from build123d import *

# Parameters (mm, degrees)
SKETCH_1_R          = 2.1
EXTRUDE_1_DEPTH     = 3
SKETCH_2_R          = 1.6
SKETCH_2_R_2        = 8
CUT_EXTRUDE_1_DEPTH = 3
CUT_EXTRUDE_2_DEPTH = 3
CUT_EXTRUDE_3_DEPTH = 3


with BuildPart() as part:
    # 草图1 → 凸台-拉伸1 (new body)
    with BuildSketch(Plane.XY):
        with BuildLine():
            Line((10, 0), (140, 0))
            ThreePointArc((140, 0), (147.071067812, -2.928932188), (150, -10))
            Line((150, -10), (150, -70))
            ThreePointArc((150, -70), (147.071067812, -77.071067812), (140, -80))
            Line((140, -80), (10, -80))
            ThreePointArc((10, -80), (2.928932188, -77.071067812), (0, -70))
            Line((0, -70), (0, -10))
            ThreePointArc((0, -10), (2.928932188, -2.928932188), (10, 0))
        make_face()
        with Locations((8, -8)):
            Circle(SKETCH_1_R, mode=Mode.SUBTRACT)
        with Locations(Location((8, -72, 0), (0, 0, 180))):
            Circle(SKETCH_1_R, mode=Mode.SUBTRACT)
        with Locations((142, -72)):
            Circle(SKETCH_1_R, mode=Mode.SUBTRACT)
        with Locations(Location((142, -8, 0), (0, 0, 180))):
            Circle(SKETCH_1_R, mode=Mode.SUBTRACT)
    extrude(amount=EXTRUDE_1_DEPTH)

    # 草图2 → 切除-拉伸1 (cut)
    with BuildSketch(Plane.XY.offset(3)):
        with Locations((52, -17)):
            Circle(SKETCH_2_R)
        with Locations((98, -17)):
            Circle(SKETCH_2_R)
        with Locations((98, -63)):
            Circle(SKETCH_2_R)
        with Locations((52, -63)):
            Circle(SKETCH_2_R)
        with Locations((75, -40)):
            Circle(SKETCH_2_R_2)
        with BuildLine():
            ThreePointArc((87.02081528, -27.97918472), (75, -23), (62.97918472, -27.97918472))
            ThreePointArc((62.97918472, -27.97918472), (62.97918472, -30.807611845), (65.807611845, -30.807611845))
            ThreePointArc((65.807611845, -30.807611845), (75, -27), (84.192388155, -30.807611845))
            ThreePointArc((84.192388155, -30.807611845), (87.02081528, -30.807611845), (87.02081528, -27.97918472))
        make_face()
        with BuildLine():
            ThreePointArc((87.02081528, -52.02081528), (75, -57), (62.97918472, -52.02081528))
            ThreePointArc((62.97918472, -52.02081528), (62.97918472, -49.192388155), (65.807611845, -49.192388155))
            ThreePointArc((65.807611845, -49.192388155), (75, -53), (84.192388155, -49.192388155))
            ThreePointArc((84.192388155, -49.192388155), (87.02081528, -49.192388155), (87.02081528, -52.02081528))
        make_face()
    extrude(amount=-CUT_EXTRUDE_1_DEPTH, mode=Mode.SUBTRACT)

    # 草图3 → 切除-拉伸2 (cut)
    with BuildSketch(Plane.XY.offset(3)):
        with BuildLine():
            Line((128, -22.5), (128, -57.5))
            ThreePointArc((128, -57.5), (123, -62.5), (118, -57.5))
            Line((118, -57.5), (118, -22.5))
            ThreePointArc((118, -22.5), (123, -17.5), (128, -22.5))
        make_face()
        with BuildLine():
            Line((22, -22.5), (22, -57.5))
            ThreePointArc((22, -57.5), (27, -62.5), (32, -57.5))
            Line((32, -57.5), (32, -22.5))
            ThreePointArc((32, -22.5), (27, -17.5), (22, -22.5))
        make_face()
        with BuildLine():
            ThreePointArc((99.574561329, -57.207293091), (105, -40), (99.574561329, -22.792706909))
            ThreePointArc((99.574561329, -22.792706909), (92.610918925, -21.56482887), (91.383040886, -28.528471273))
            ThreePointArc((91.383040886, -28.528471273), (95, -40), (91.383040886, -51.471528727))
            ThreePointArc((91.383040886, -51.471528727), (92.610918925, -58.43517113), (99.574561329, -57.207293091))
        make_face()
        with BuildLine():
            ThreePointArc((50.425438671, -57.207293091), (45, -40), (50.425438671, -22.792706909))
            ThreePointArc((50.425438671, -22.792706909), (57.389081075, -21.56482887), (58.616959114, -28.528471273))
            ThreePointArc((58.616959114, -28.528471273), (55, -40), (58.616959114, -51.471528727))
            ThreePointArc((58.616959114, -51.471528727), (57.389081075, -58.43517113), (50.425438671, -57.207293091))
        make_face()
    extrude(amount=-CUT_EXTRUDE_2_DEPTH, mode=Mode.SUBTRACT)

    # 草图4 → 切除-拉伸3 (cut)
    with BuildSketch(Plane(origin=(0, 0, 0), x_dir=(-1, 0, 0), z_dir=(0, 0, -1))):
        with BuildLine():
            Line((-97.5, -4), (-52.5, -4))
            ThreePointArc((-52.5, -4), (-48.5, -8), (-52.5, -12))
            Line((-52.5, -12), (-97.5, -12))
            ThreePointArc((-97.5, -12), (-101.5, -8), (-97.5, -4))
        make_face()
        with BuildLine():
            Line((-97.5, -76), (-52.5, -76))
            ThreePointArc((-52.5, -76), (-48.5, -72), (-52.5, -68))
            Line((-52.5, -68), (-97.5, -68))
            ThreePointArc((-97.5, -68), (-101.5, -72), (-97.5, -76))
        make_face()
    extrude(amount=-CUT_EXTRUDE_3_DEPTH, mode=Mode.SUBTRACT)


solid = part.part
Read the model definition and answer for the solid it produces. Units are mm, in the model's axes. Round coordinates to 2 decimals unless told otherwise and drop trailing zeros. Write each loop counter-clockwise with the first axis right and the second up, starting at its lowest first coordinate (ties: lowest second). Pieces come first, ordered by that corner, then holes.
Q1. A flat-ended cylindrical pin translates along its axis: P1, Ø3.5, axis at x = 52, y = -63, coming from the +Z side. Find the tip coordinate at first contact, or state that the pin passes through.
Values:
P1: stops at z = 3
Q2. Straight lines are drawn through the part: line 1 (Y direction, x = 75, z = 2.15); line 2 (Y direction, x = 8.5, z = 0.35); line 3 (X direction, y = -37, z = 2.65). For each, find the intervals that lie inside material, in ascending order.
Values:
line 1: y = -80 to -76, -68 to -57, -53 to -48, -32 to -27, -23 to -12, -4 to 0
line 2: y = -79.89 to -74.04, -69.96 to -10.04, -5.96 to -0.11
line 3: x = 0 to 22, 32 to 45.15, 55.23 to 67.58, 82.42 to 94.77, 104.85 to 118, 128 to 150
Q3. Find section C-C on z = 1.6. State how many separate pieces and enclosed holes the cut face has, and give its area (3 significant figures).
Values:
separate pieces: 1
enclosed holes: 17
area: 8,970 mm2
Q4. Find section A-A on x = 123. Determine the outline of the cut face in (y, z).
Values:
outline: (-80, 0) - (-62.5, 0) - (-62.5, 3) - (-80, 3) - close; (-17.5, 0) - (0, 0) - (0, 3) - (-17.5, 3) - close
Q5. Find section B-B on x = 69. Determine the outline of the cut face in (y, z), and give its area (3 significant figures).
Values:
outline: (-80, 0) - (-76, 0) - (-76, 3) - (-80, 3) - close; (-68, 0) - (-55.91, 0) - (-55.91, 3) - (-68, 3) - close; (-51.53, 0) - (-45.29, 0) - (-45.29, 3) - (-51.53, 3) - close; (-34.71, 0) - (-28.47, 0) - (-28.47, 3) - (-34.71, 3) - close; (-24.09, 0) - (-12, 0) - (-12, 3) - (-24.09, 3) - close; (-4, 0) - (0, 0) - (0, 3) - (-4, 3) - close
area: 134 mm2
Q6. The mould has two halves that part along Y. Classify faces 1 (the face through (75, -53, 2)), 2 (the face through (76, -80, 1)), 3 (the face through (76, -31, 3)): released by +Y, released by -Y, zero draft, split by the parting line, or undercut.
Values:
face 1: undercut
face 2: released by -Y
face 3: zero draft
